Answer from the drawing. Dimensions are ordinates in mm from the lowest x, y and z of the part. A direction names the side the tool comes from. Give positions to 0.01 mm unless a question says otherwise; leave off trailing zeros. Write each loop counter-clockwise with the first axis right and the second up, starting at its lowest first coordinate (ties: lowest second). Pieces come first, ordered by that corner, then holes.
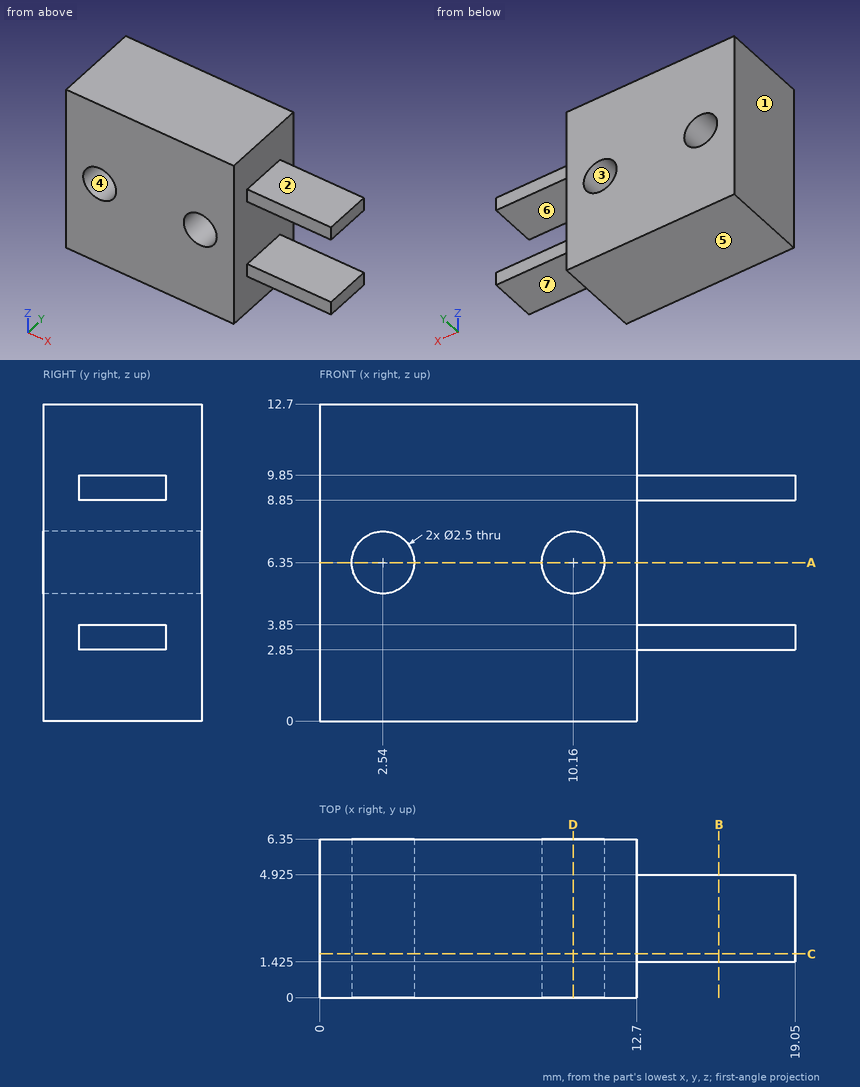
Item 1: Each of these flat-tipped pins is pushed along its axis until it touches: P1, Ø0.5, axis at x = 15.5, z = 3.5, coming from the +Y side (3 decimals); P2, Ø2, axis at x = 2.54, z = 6.35, coming from the +Y side; P3, Ø1.9, axis at y = 4, z = 5.5, coming from the +X side; P4, Ø3, axis at x = 15, y = 3, coming from the +Z side. Where does it stop, or does it pass through?
Conclusion:
P1: stops at y = 4.925
P2: passes through
P3: stops at x = 12.7
P4: stops at z = 9.85
Item 2: Consider probe 1 along X at (y, z) = (4.5, 6.35); probe 2 along Z at (x, y) = (17.75, 2.5); probe 3 along Z at (x, y) = (10.16, 5). Determine where each line is inside the solid, lowest interval first.
Conclusion:
probe 1: x = 0 to 1.29, 3.79 to 8.91, 11.41 to 12.7
probe 2: z = 2.85 to 3.85, 8.85 to 9.85
probe 3: z = 0 to 5.1, 7.6 to 12.7
Item 3: A cutting plane is placed at B-B, the plane x = 16. Give the vertices of the cut face in (y, z) (3 decimals).
Conclusion:
outline: (1.425, 2.85) - (4.925, 2.85) - (4.925, 3.85) - (1.425, 3.85) - close; (1.425, 8.85) - (4.925, 8.85) - (4.925, 9.85) - (1.425, 9.85) - close
Item 4: A cutting plane is placed at D-D, the plane x = 10.16. Give the vertices of the cut face in (y, z), plus the area to 3 significant figures.
Conclusion:
outline: (0, 0) - (6.35, 0) - (6.35, 5.1) - (0, 5.1) - close; (0, 7.6) - (6.35, 7.6) - (6.35, 12.7) - (0, 12.7) - close
area: 64.8 mm2
Item 5: A cutting plane is placed at A-A, the plane z = 6.35. Give the vertices of the cut face in (x, y), plus the area to 3 significant figures.
Conclusion:
outline: (0, 0) - (1.29, 0) - (1.29, 6.35) - (0, 6.35) - close; (3.79, 0) - (8.91, 0) - (8.91, 6.35) - (3.79, 6.35) - close; (11.41, 0) - (12.7, 0) - (12.7, 6.35) - (11.41, 6.35) - close
area: 48.9 mm2
Item 6: A cutting plane is placed at C-C, the plane y = 1.75. Give the vertices of the cut face in (x, z).
Conclusion:
outline: (0, 0) - (12.7, 0) - (12.7, 2.85) - (19.05, 2.85) - (19.05, 3.85) - (12.7, 3.85) - (12.7, 8.85) - (19.05, 8.85) - (19.05, 9.85) - (12.7, 9.85) - (12.7, 12.7) - (0, 12.7) - close; hole circle Ø2.5 at (2.54, 6.35); hole circle Ø2.5 at (10.16, 6.35)
Item 7: Determine the mould class of the marked faces 1, 2, 3 and 4 for opening direction X: pulls with the +X half, pulls with the -X half, needs draft (parallel to the pull), parting line crosses it, or undercut.
Conclusion:
face 1: pulls with the -X half
face 2: needs draft
face 3: undercut
face 4: undercut
Item 8: Which of the six approach directions +Z, -Z, +X, -X, +Y, -Y give full straight-line access (tool end or side, diameter ignored) to the marked faces 5, 6 and 7?
Conclusion:
face 5: -Z, +X, -X, +Y, -Y
face 6: +X, +Y, -Y
face 7: -Z, +X, +Y, -Y
